Read the model definition and answer for the solid it produces. Units are mm, in the model's axes. Face numbers are marked on the shaded views. A direction names the side the tool comes from. Coordinates: 2 decimals unless noted, no trailing zeros. Order: outer loops, then holes, each group sorted by start corner. A loop starts at its lowest first (then second) coordinate and runs counter-clockwise, first axis right, second up.
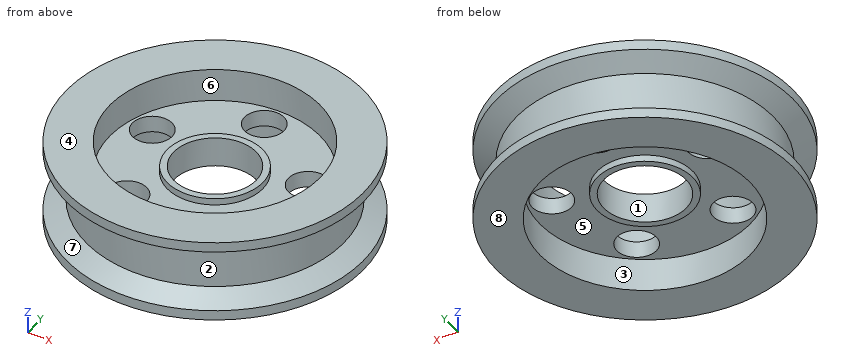
from build123d import *

# Parameters (mm, degrees)
SKETCH1_R                = 45
SKETCH1_R_2              = 12.5
BOSS_EXTRUDE1_DEPTH      = 12.5
SKETCH2_R                = 31.875
CUT_EXTRUDE1_DEPTH       = 10
SKETCH3_R                = 6
CUT_EXTRUDE2_DEPTH       = 66.383484153
CIRPATTERN1_COUNT        = 5
BOSS_EXTRUDE2_DEPTH      = 2
BOSS_EXTRUDE2_DEPTH_BACK = 7
SKETCH4_R                = 14.5
SKETCH4_R_2              = 12.5


with BuildPart() as part:
    # Sketch1 → Boss-Extrude1 (new, symmetric)
    with BuildSketch(Plane.XY):
        Circle(SKETCH1_R)
        Circle(SKETCH1_R_2, mode=Mode.SUBTRACT)
    extrude(amount=BOSS_EXTRUDE1_DEPTH, both=True)

    # Sketch2 → Cut-Extrude1 (cut)
    with BuildSketch(Plane.XY.offset(12.5)):
        Circle(SKETCH2_R)
    cut_extrude1 = extrude(amount=-CUT_EXTRUDE1_DEPTH, mode=Mode.SUBTRACT)

    # Mirror1: Cut-Extrude1 across plane
    add(cut_extrude1.mirror(Plane.XY), mode=Mode.SUBTRACT)

    # Sketch3 → Cut-Extrude2 (cut, through all)
    with BuildSketch(Plane.XY.offset(2.5)):
        with Locations((0, 25)):
            Circle(SKETCH3_R)
    cut_extrude2 = extrude(amount=-CUT_EXTRUDE2_DEPTH, mode=Mode.SUBTRACT)

    # CirPattern1: Cut-Extrude2 ×5 about axis
    cirpattern1_axis = Axis((0, 0, 0), (0, 0, 1))
    for i in range(1, CIRPATTERN1_COUNT):
        add(cut_extrude2.rotate(cirpattern1_axis, i * 360 / CIRPATTERN1_COUNT), mode=Mode.SUBTRACT)

    # Sketch4 → Boss-Extrude2 (add, two sides: drawn at the far end of the back side and taken through both)
    with BuildSketch(Plane.XY.offset(2.5).offset(-BOSS_EXTRUDE2_DEPTH_BACK)):
        Circle(SKETCH4_R)
        Circle(SKETCH4_R_2, mode=Mode.SUBTRACT)
    extrude(amount=BOSS_EXTRUDE2_DEPTH + BOSS_EXTRUDE2_DEPTH_BACK)

    # Sketch5 → Cut-Revolve1 (revolve, cut)
    with BuildSketch(Plane(origin=(0, 0, 0), x_dir=(1, 0, 0), z_dir=(0, 1, 0))):
        Polygon((45, 9.5), (39, 6.035898385), (39, -6.035898385), (45, -9.5), align=None)
    revolve(axis=Axis((0, 0, 0), (0, 0, -1)), mode=Mode.SUBTRACT)


solid = part.part
Q1. The part is cut by section B-B, the plane x = 0. State how many separate pieces and enclosed holes the cut face has, then the cut area to 3 significant figures.
Q2. Determine the mould class of the marked faces 1, 2, 3 and 4 for opening direction X: +X half, -X half, draft (parallel to the pull), parting line (faces both ways), or undercut.
Q3. Each of these flat-tipped pins is pushed along its axis until it touches: P1, Ø23, axis at x = 0, y = -3, coming from the +Z side; P2, Ø12, axis at x = 14, y = -14, coming from the -Z side; P3, Ø8, axis at y = -18.5, z = 7, coming from the -X side. Where does it stop, or does it pass through?
Q4. The part is cut by section C-C, the plane z = -7.25. Determine the outline of the cut face in (x, y) (3 decimals), then the cut area to 3 significant figures.
Q5. Straight lines are drawn through the part: L1, parallel to Y at x = 0, z = -0.5; L2, parallel to Y at x = 0, z = -10 (3 decimals); L3, parallel to X at y = -19.5, z = 2.25 (3 decimals). For each, find the intervals that lie inside material, in ascending order.
Q6. Which of the six approach directions +Z, -Z, +X, -X, +Y, -Y give full straight-line access (tool end or side, diameter ignored) to the marked faces 5, 6, 7 and 8?
Computed values:
1. separate pieces: 3
1. enclosed holes: 0
1. area: 620 mm2
2. face 1: undercut
2. face 2: parting line
2. face 3: undercut
2. face 4: draft
3. P1: stops at z = 4.5
3. P2: stops at z = -4.5
3. P3: stops at x = -42.29
4. outline: circle Ø82.206 at (0, 0); hole circle Ø63.75 at (0, 0)
4. area: 2,120 mm2
5. L1: y = -39 to -12.5, 12.5 to 19, 31 to 39
5. L2: y = -45 to -31.875, 31.875 to 45
5. L3: x = -33.775 to -20.651, -8.739 to 8.739, 20.651 to 33.775
6. face 5: -Z
6. face 6: +Z
6. face 7: none
6. face 8: -Z, +X, -X, +Y, -Y
